The drawing under review shows one solid part. Ordinate dimensions are in mm from its lowest x, y, z. Round coordinates to 2 decimals unless told otherwise and drop trailing zeros. Order: outer loops, then holes, each group sorted by start corner. A loop starts at its lowest first (then second) coordinate and runs counter-clockwise, first axis right, second up. Notation, with made-up numbers: (2, 49.5) - (23, 49.5) arc R14 ccw to (23, 57.5) - close; hole circle Ø3 at (14.5, 60). An arc over 180 degrees is marked (long way). One line per question, with ' | ' between items.
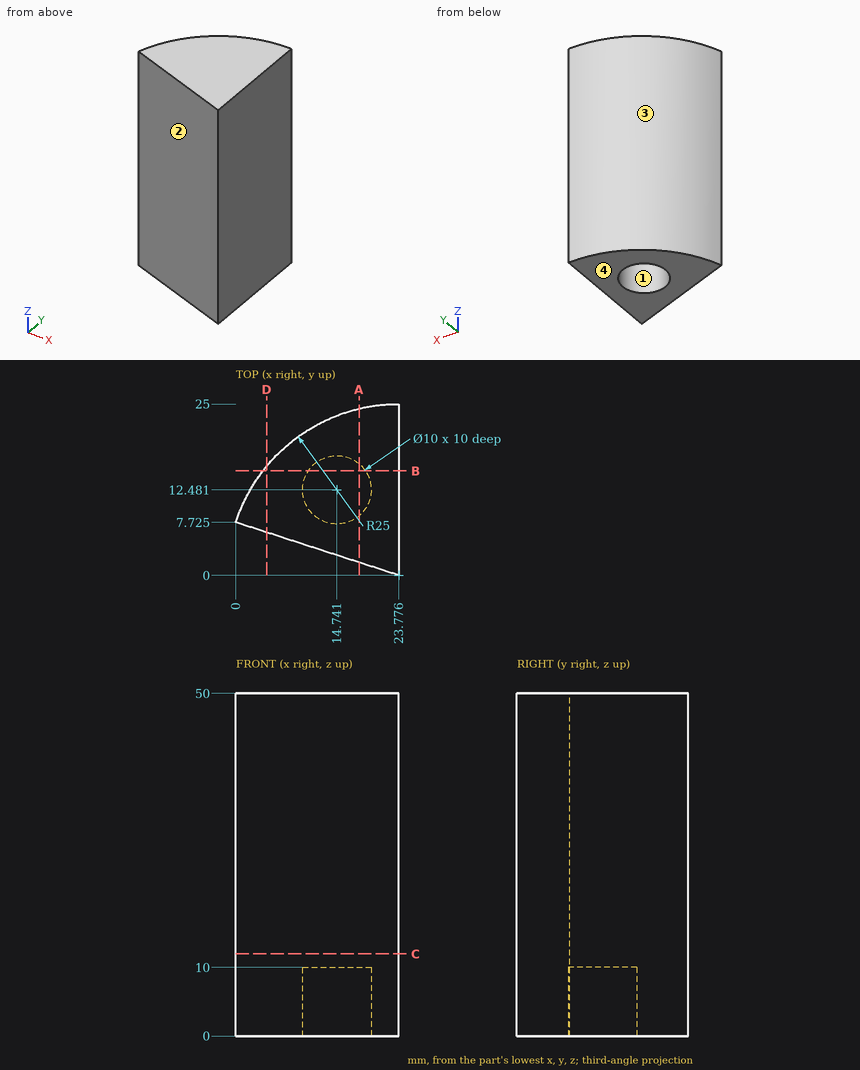
(1) Insertion check: pin 1 (5 mm diameter, centred on x = 13, y = 12, fed in from -Z); pin 2 (12 mm diameter, centred on x = 4, z = 44, fed in from -Y); pin 3 (4 mm diameter, centred on x = 17, z = 15, fed in from +Y). Each pin has a flat end and moves straight along its axis. Give the tip position at first contact, or say it passes through.
Output values:
pin 1: z = 10 | pin 2: y = 4.48 | pin 3: y = 24.54
(2) We need section A-A on x = 18. State the section outline as (y, z) points, plus the area to 3 significant figures.
Output values:
outline: (1.88, 0) - (8.69, 0) - (8.69, 10) - (16.27, 10) - (16.27, 0) - (24.32, 0) - (24.32, 50) - (1.88, 50) - close | area: 1,050 mm^2
(3) We need section D-D on x = 4.5. State the section outline as (y, z) points.
Output values:
outline: (6.26, 0) - (15.92, 0) - (15.92, 50) - (6.26, 50) - close
(4) For probe 1 along Z at (x, y) = (17, 15.5); probe 2 along Y at (x, z) = (20, 5.5); probe 3 along Y at (x, z) = (1.25, 20) (1 decimal), list the stretches that pass through material, from the lowest coordinate up. Write a range as [from, to].
Output values:
probe 1: [10, 50] | probe 2: [1.23, 24.71] | probe 3: [7.3, 10.8]
(5) We need section B-B on y = 15.25. State the section outline as (x, z) points (1 decimal).
Output values:
outline: (4, 0) - (10.6, 0) - (10.6, 10) - (18.9, 10) - (18.9, 0) - (23.8, 0) - (23.8, 50) - (4, 50) - close
(6) We need section C-C on z = 12. State the section outline as (x, y) points (1 decimal).
Output values:
outline: (0, 7.7) - (23.8, 0) - (23.8, 25) arc R25 ccw to start
(7) Mouldability with a two-part tool opening along Y and no side actions: class the marked faces 1, 2, 3 and 4 as released by +Y, released by -Y, zero draft, split by the parting line, or undercut.
Output values:
face 1: undercut | face 2: released by -Y | face 3: released by +Y | face 4: zero draft
